The listing builds one solid part. Answer for the finished solid, in the listing's coordinates (mm). Face numbers are marked on the shaded views. A direction names the side the tool comes from. Round coordinates to 2 decimals unless told otherwise and drop trailing zeros. Write each loop counter-clockwise with the first axis right and the second up, starting at its lowest first coordinate (ties: lowest second). Pieces come first, ordered by that corner, then holes.
Item 1: Find section A-A on x = 0. Give the vertices of the cut face in (y, z), then the cut area to 3 significant figures.
Item 2: Each of these flat-tipped pins is pushed along its axis until it touches: pin 1 (0.8 mm diameter, centred on y = -1, z = -2, fed in from -X); pin 2 (1.1 mm diameter, centred on x = 1, z = -2, fed in from +Y); pin 3 (0.8 mm diameter, centred on x = -1.5, z = -2, fed in from -Y). Where does it stop, or does it pass through?
Item 3: A tool of negligible diameter and unlimited length cuts with its end or side. For the marked faces 1 and 2, from which of +Z, -Z, +X, -X, +Y, -Y can it reach the whole face along a straight path? Write none if from no direction.
Item 4: Find the intervals of material crossed by probe 1 along Y at (x, z) = (0, 13.5); probe 2 along Z at (x, y) = (0, -0.75); probe 3 along Z at (x, y) = (0, -1.75), in increasing order.
Item 5: Find section C-C on z = 20.25. Give the vertices of the cut face in (x, y).
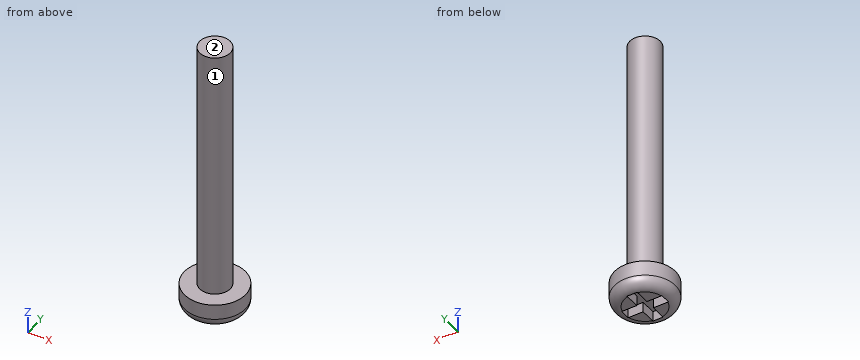
Autodesk Inventor part; units mm, degrees
ref_plane "YZ Plane" through (0, 0, 0) normal (1, 0, 0) x (0, 1, 0)
ref_plane "XZ Plane" through (0, 0, 0) normal (0, 1, 0) x (-1, 0, 0)
ref_plane "XY Plane" through (0, 0, 0) normal (0, 0, 1) x (1, 0, 0)
sketch "Sketch1" plane through (0, 0, 0) normal (0, 0, 1) x (1, 0, 0)
  circle A0 centre (0, 0) radius 1.5
  circle A1 centre (0, 0) radius 3
  dimension "d0" = 3
  dimension "d1" = 6
extrude "Extrusion1" add sketch "Sketch1" along normal blind 25 contours A0
sketch "Sketch2" plane through (0, 0, 0) normal (0, 0, -1) x (-1, 0, 0)
  point P0 (0, 0)
extrude "Extrusion2" add sketch "Sketch1" against normal blind 2.5 contours A0 | A1
thread "Thread1"
sketch "Sketch3" plane through (0, 0, -2.5) normal (0, 0, -1) x (-1, 0, 0)
  point P0 (0, 0)
sketch "Sketch4" plane through (0, 0, -2.5) normal (0, 0, -1) x (-1, 0, 0)
  line L0 (-0.5, -2) -> (0.5, -2)
  line L1 (0.5, -2) -> (0.5, 2)
  line L2 (0.5, 2) -> (-0.5, 2)
  line L3 (-0.5, 2) -> (-0.5, -2)
  circle A0 centre (0, 0) radius 1.5
  line L4 (-0.5, -2) -> (0.5, 2) construction
  line L5 (0.5, -2) -> (-0.5, 2) construction
  line L6 (-2, -0.5) -> (2, -0.5)
  line L7 (2, -0.5) -> (2, 0.5)
  line L8 (2, 0.5) -> (-2, 0.5)
  line L9 (-2, 0.5) -> (-2, -0.5)
  circle A1 centre (0, 0) radius 3
  line L10 (-2, -0.5) -> (2, 0.5) construction
  line L11 (2, -0.5) -> (-2, 0.5) construction
  point P0 (-0.5, 0.5)
  point P1 (-0.5, -0.5)
  point P2 (0.5, -0.5)
  point P3 (0.5, 0.5)
  dimension "d8" = 1
  dimension "d9" = 4
  dimension "d10" = 4
  dimension "d11" = 1
extrude "Extrusion3" cut sketch "Sketch4" against normal blind 1 contours L3 A0 L1 L0 | L3 L6 L1 A0 | L6 A0 L8 L3 | L3 L8 L1 L6 | L6 L9 L8 A0 | L1 L8 A0 L6 | A0 L8 L7 L6 | L3 A0 L1 L8 | L3 L2 L1 A0
fillet "Fillet1" radius 1 1 edges at (-3, 0, -2.5)
properties part number "16x2.5 Bolt"
Check values:
1. outline: (-3, -1.5) arc R1 ccw to (-2, -2.5) - (-2, -1.5) - (2, -1.5) - (2, -2.5) arc R1 ccw to (3, -1.5) - (3, 0) - (1.5, 0) - (1.5, 25) - (-1.5, 25) - (-1.5, 0) - (-3, 0) - close
1. area: 85.6 mm2
2. pin 1: stops at x = -2.89
2. pin 2: stops at y = 2.93
2. pin 3: stops at y = -2.72
3. face 1: +Z
3. face 2: +Z, +X, -X, +Y, -Y
4. probe 1: y = -1.5 to 1.5
4. probe 2: z = -1.5 to 25
4. probe 3: z = -1.5 to 0
5. outline: circle Ø3 at (0, 0)
